Can you work these out from the drawing? Everything is in mm from the part's minimum corner. A direction names the side the tool comes from. Round coordinates to 2 decimals unless told otherwise and drop trailing zeros. Write each loop counter-clockwise with the first axis right and the second up, starting at its lowest first coordinate (ties: lowest second). Pieces come first, ordered by that corner, then holes. Notation, with made-up numbers: (-29.75, 61.5) -> (17.25, 61.5) arc R31 cw to (17.25, 98.5) -> close; hole circle Ø5 at (-9.75, 66.25). An arc over 180 degrees is marked (long way). Answer as CSV lines item,"result".
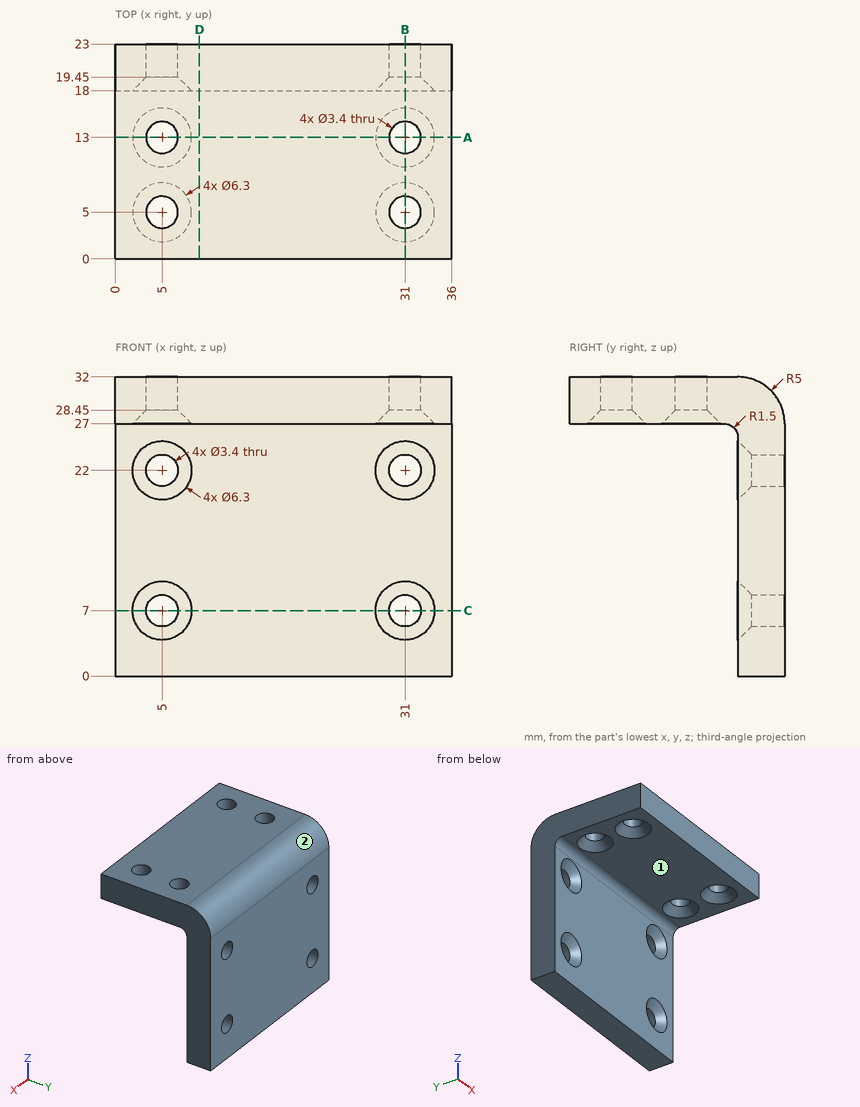
Item 1: I need wall thicknesses on L1, parallel to X at y = 5, z = 30.25; L2, parallel to Z at x = 5, y = 21.55; L3, parallel to Y at x = 5, z = 29.8. Which ranges of each line are inside material? Lowest first, please.
Results found:
L1,"x = 0 to 3.3, 6.7 to 29.3, 32.7 to 36"
L2,"z = 0 to 5.3, 8.7 to 20.3, 23.7 to 30.52"
L3,"y = 0 to 3.3, 6.7 to 11.3, 14.7 to 22.14"
Item 2: For the marked faces 1 and 2, which set-ups out of +Z, -Z, +X, -X, +Y, -Y let a thin tool reach every point of the face, with its end or its side?
Results found:
face 1,"-Z, +X, -X, -Y"
face 2,"+Z, +X, -X, +Y"
Item 3: Suppose I cut it at D-D, the plane x = 9. List the corners of the cut face in (y, z) for me.
Results found:
outline,"(0, 27) -> (16.5, 27) arc R1.5 cw to (18, 25.5) -> (18, 0) -> (23, 0) -> (23, 27) arc R5 ccw to (18, 32) -> (0, 32) -> close"
Item 4: Will these pins go through, and if not, where does the flat tip stop? pin 1 (5.5 mm diameter, centred on x = 5, z = 7, fed in from +Y); pin 2 (8 mm diameter, centred on x = 17.5, y = 10, fed in from -Z); pin 3 (7.5 mm diameter, centred on x = 17, z = 15.5, fed in from -Y); pin 4 (4 mm diameter, centred on x = 31, y = 5, fed in from -Z).
Results found:
pin 1,"stops at y = 23"
pin 2,"stops at z = 27"
pin 3,"stops at y = 18"
pin 4,"stops at z = 28.15"
Item 5: Suppose I cut it at A-A, the plane y = 13. List the corners of the cut face in (x, z) for me.
Results found:
outline,"(0, 27) -> (1.85, 27) -> (3.3, 28.45) -> (3.3, 32) -> (0, 32) -> close; (6.7, 28.45) -> (8.15, 27) -> (27.85, 27) -> (29.3, 28.45) -> (29.3, 32) -> (6.7, 32) -> close; (32.7, 28.45) -> (34.15, 27) -> (36, 27) -> (36, 32) -> (32.7, 32) -> close"
Item 6: Suppose I cut it at C-C, the plane z = 7. List the corners of the cut face in (x, y) for me.
Results found:
outline,"(0, 18) -> (1.85, 18) -> (3.3, 19.45) -> (3.3, 23) -> (0, 23) -> close; (6.7, 19.45) -> (8.15, 18) -> (27.85, 18) -> (29.3, 19.45) -> (29.3, 23) -> (6.7, 23) -> close; (32.7, 19.45) -> (34.15, 18) -> (36, 18) -> (36, 23) -> (32.7, 23) -> close"
Item 7: Suppose I cut it at B-B, the plane x = 31. State how many separate pieces and enclosed holes the cut face has, then the cut area to 3 significant figures.
Results found:
separate pieces,"5"
enclosed holes,"0"
area,"169 mm²"
